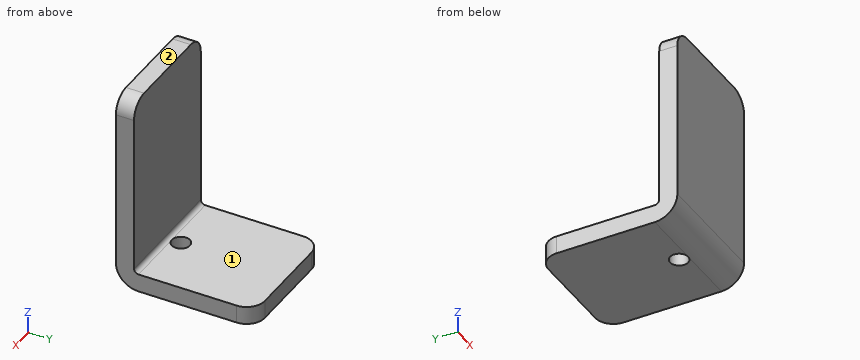
```python
from build123d import *

# Parameters (mm, degrees)
BASE_FLANGE1_DEPTH = 20
FILLET1_R          = 3
SKETCH5_R          = 1.5
CUT_EXTRUDE1_DEPTH = 44.462627624


# Sheet-metal steps are written as plain solids
with BuildPart() as part:
    # Sketch1 → Base-Flange1 (new body)
    with BuildSketch(Plane(origin=(0, 0, 0), x_dir=(0, 0, -1), z_dir=(1, 0, 0))):
        with BuildLine():
            Line((0, 0), (29.2634, 0))
            ThreePointArc((29.2634, 0), (29.784254855, 0.215745145), (30, 0.7366))
            Line((30, 0.7366), (30, 20))
            Line((30, 20), (33, 20))
            Line((33, 20), (33, 0.7366))
            ThreePointArc((33, 0.7366), (31.905575199, -1.905575199), (29.2634, -3))
            Line((29.2634, -3), (0, -3))
            Line((0, -3), (0, 0))
        make_face()
    extrude(amount=BASE_FLANGE1_DEPTH)

    # Fillet1
    fillet1_edges = [part.edges().sort_by_distance(p)[0] for p in [
        (20, -1.5, 0),
        (20, 20, -31.5),
        (0, -1.5, 0),
        (0, 20, -31.5),
    ]]
    fillet(fillet1_edges, radius=FILLET1_R)

    # Sketch5 → Cut-Extrude1 (cut, through all)
    with BuildSketch(Plane(origin=(0, 0, -33), x_dir=(-1, 0, 0), z_dir=(0, 0, -1))):
        with Locations(Location((-10, 2.2366, 0), (0, 0, 270))):
            Circle(SKETCH5_R)
    extrude(amount=-CUT_EXTRUDE1_DEPTH, mode=Mode.SUBTRACT)


solid = part.part
```
Verification items for the finished model (mm, model axes). Face numbers are marked on the shaded views. A direction names the side the tool comes from. Give positions to 0.01 mm unless a question says otherwise; leave off trailing zeros. Loops run counter-clockwise (first coordinate to the right, second up) from the corner with the lowest first, then second, coordinate; pieces in that order, holes last.
1. Section check D-D, the plane x = 18.25. Enter the section's corners in (y, z), then the cut area to 3 significant figures.
2. Go/stop test with flat-tipped pins: pin 1 Ø4 at (x, z) = (13, -9.5) entering from +Y; pin 2 Ø1.5 at (x, y) = (13.5, 15.5) entering from +Z; pin 3 Ø4 at (y, z) = (12.5, -29.5) entering from +X; pin 4 Ø4 at (x, y) = (10, 2.24) entering from +Z. Record where each tip stops, or that it passes through.
3. Section check C-C, the plane z = -17. Enter the section's corners in (x, y), then the cut area to 3 significant figures.
4. Section check B-B, the plane y = 10.5. Enter the section's corners in (x, z), then the cut area to 3 significant figures.
5. Thickness scan on line 1 (Z direction, x = 13.25, y = 4); line 2 (Y direction, x = 16.25, z = -7); line 3 (Y direction, x = 10, z = -30.6). Record the ranges inside material, lowest first.
6. Section check A-A, the plane x = 5.75. Enter the section's corners in (y, z), then the cut area to 3 significant figures.
7. Set-up check for the marked faces 1 and 2: record each of +Z, -Z, +X, -X, +Y, -Y from which the full face is reachable in a straight line by a thin tool's end or side.
Geometry says:
1. outline: (-3, -29.26) arc R3.74 ccw to (0.74, -33) - (19.73, -33) - (19.73, -30) - (0.74, -30) arc R0.74 cw to (0, -29.26) - (0, -0.27) - (-3, -0.27) - close
1. area: 154 mm2
2. pin 1: stops at y = 0
2. pin 2: stops at z = -30
2. pin 3: stops at x = 20
2. pin 4: stops at z = -29.81
3. outline: (0, -3) - (20, -3) - (20, 0) - (0, 0) - close
3. area: 60.0 mm2
4. outline: (0, -33) - (20, -33) - (20, -30) - (0, -30) - close
4. area: 60.0 mm2
5. line 1: z = -33 to -30
5. line 2: y = -3 to 0
5. line 3: y = -2.75 to 0.74, 3.74 to 20
6. outline: (-3, -29.26) arc R3.74 ccw to (0.74, -33) - (20, -33) - (20, -30) - (0.74, -30) arc R0.74 cw to (0, -29.26) - (0, 0) - (-3, 0) - close
6. area: 156 mm2
7. face 1: +Z, +X, -X, +Y
7. face 2: +Z, +X, -X, +Y, -Y
